```python
from build123d import *

# Parameters (mm, degrees)
F0_W     = 160
F0_H     = 180
F0_R     = 4.25
F0_R_2   = 5
F1_DEPTH = 8
F2_SIZE  = 10


with BuildPart() as f1:
    # F0 (on Front) → F1 (new body)
    with BuildSketch(Plane.XZ):
        Rectangle(F0_W, F0_H)
        with Locations((-60, -49)):
            Circle(F0_R, mode=Mode.SUBTRACT)
        with Locations((-18.25, -72)):
            Circle(F0_R_2, mode=Mode.SUBTRACT)
        with Locations((18.25, -72)):
            Circle(F0_R_2, mode=Mode.SUBTRACT)
        with Locations((60, -49)):
            Circle(F0_R, mode=Mode.SUBTRACT)
        with Locations((-60, 34)):
            Circle(F0_R, mode=Mode.SUBTRACT)
        with Locations((12, 20)):
            Circle(F0_R, mode=Mode.SUBTRACT)
        with Locations((60, 34)):
            Circle(F0_R, mode=Mode.SUBTRACT)
        with Locations((12, 64.5)):
            Circle(F0_R, mode=Mode.SUBTRACT)
    extrude(amount=F1_DEPTH)

    # F2
    f2_edges = [f1.edges().sort_by_distance(p)[0] for p in [
        (-80, -4, 90),
        (80, -4, 90),
        (80, -4, -90),
        (-80, -4, -90),
    ]]
    chamfer(f2_edges, length=F2_SIZE)


solid = f1.part
```
Verification items for the finished model (mm, model axes). Round coordinates to 2 decimals unless told otherwise and drop trailing zeros. Write each loop counter-clockwise with the first axis right and the second up, starting at its lowest first coordinate (ties: lowest second). Pieces come first, ordered by that corner, then holes. Notation, with made-up numbers: (-24, -9) - (4, -9) arc R10 ccw to (4, 4) - close; hole circle Ø10 at (-40, 16.5). An arc over 180 degrees is marked (long way). Answer as a JSON object with one key per item and string values. Group by question number.
Q1. Thickness scan on line 1 (Z direction, x = 60, y = -4.25); line 2 (Z direction, x = 12, y = -1.5); line 3 (Z direction, x = -18, y = -1.5). Record the ranges inside material, lowest first.
Q2. Section check C-C, the plane z = 20. Enter the section's corners in (x, y).
Q3. Mould release check, pull along Z, two halves, no side actions. Record for faces 1 (the flat face through (-80, -4, -1)), 2 (the cylindrical face through (11.08, -3.94, 60.35)), 3 (the flat face through (-1, -4, 90)): released by +Z, released by -Z, zero draft, split by the parting line, or undercut.
Q4. Section check A-A, the plane z = -49. Enter the section's corners in (x, y), plus the area to 3 significant figures.
Q5. Go/stop test with a flat-tipped pin: pin 1 Ø13.5 at (x, z) = (60, 34) entering from +Y. Record where the tip stops, or that it passes through.
Q6. Section check D-D, the plane y = -6.25. Give the number of separate pieces and of enclosed holes in the cut face, plus the area to 3 significant figures.
Q7. Section check B-B, the plane x = 18.25. Enter the section's corners in (y, z).
Found:
{
 "1": {"line 1": "z = -90 to -53.25, -44.75 to 29.75, 38.25 to 90", "line 2": "z = -90 to 15.75, 24.25 to 60.25, 68.75 to 90", "line 3": "z = -90 to -76.99, -67.01 to 90"},
 "2": {"outline": "(-80, -8) - (7.75, -8) - (7.75, 0) - (-80, 0) - close; (16.25, -8) - (80, -8) - (80, 0) - (16.25, 0) - close"},
 "3": {"face 1": "zero draft", "face 2": "undercut", "face 3": "released by +Z"},
 "4": {"outline": "(-80, -8) - (-64.25, -8) - (-64.25, 0) - (-80, 0) - close; (-55.75, -8) - (55.75, -8) - (55.75, 0) - (-55.75, 0) - close; (64.25, -8) - (80, -8) - (80, 0) - (64.25, 0) - close", "area": "1,140 mm^2"},
 "5": {"pin 1": "stops at y = 0"},
 "6": {"separate pieces": "1", "enclosed holes": "8", "area": "28,100 mm^2"},
 "7": {"outline": "(-8, -90) - (0, -90) - (0, -77) - (-8, -77) - close; (-8, -67) - (0, -67) - (0, 90) - (-8, 90) - close"}
}
